Work out the finished part from the listing and answer in its coordinate system (mm). Face numbers are marked on the shaded views. Coordinates: 2 decimals unless noted, no trailing zeros. Write each loop counter-clockwise with the first axis right and the second up, starting at its lowest first coordinate (ties: lowest second). Pieces come first, ordered by that corner, then holes. Notation, with made-up numbers: (-21, 3) - (8, 3) arc R24 ccw to (8, 15) - close; hole circle Ø9 at (66, 36.25). An arc over 180 degrees is marked (long way). Use one line per item in the form item = value. Start each with the question number.
Item 1: Consider probe 1 along Z at (x, y) = (45.25, 0); probe 2 along Z at (x, y) = (21.5, 0); probe 3 along X at (y, z) = (7, 34). Determine where each line is inside the solid, lowest interval first.
Item 2: A cutting plane is placed at A-A (z = -2). Write down the section's boundary in (x, y), then the cut area to 3 significant figures.
Item 3: A cutting plane is placed at D-D (y = 8). Write down the section's boundary in (x, z).
Item 4: A cutting plane is placed at C-C (x = -40). Write down the section's boundary in (y, z).
Item 5: A cutting plane is placed at B-B (y = 0). Write down the section's boundary in (x, z), then the cut area to 3 significant figures.
Item 6: Determine the mould class of the marked faces 1, 2 and 3 for opening direction X: released by +X, released by -X, zero draft, split by the parting line, or undercut.
Item 7: Given pin 1 (3 mm diameter, centred on x = 37, z = 7, fed in from -Y); pin 2 (1.5 mm diameter, centred on x = -20, z = 0, fed in from +Y); pin 3 (5 mm diameter, centred on x = 15, y = 10, fed in from +Z); pin 4 (8 mm diameter, centred on y = 0, z = 34.76, fed in from -X) (1 decimal), each flat-ended and moving along its own axis, determine where each tip first touches the part or whether it passes through.
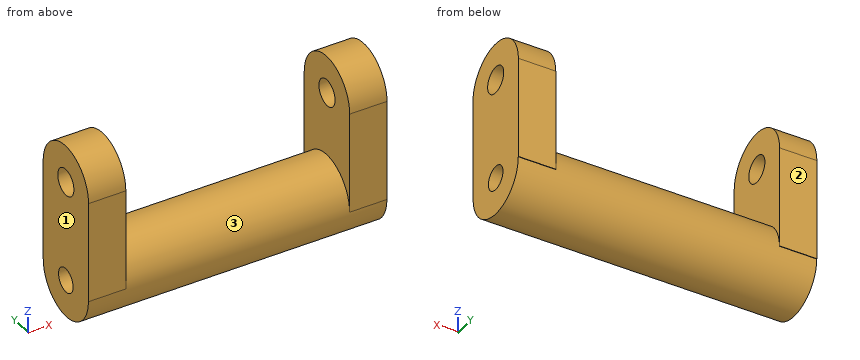
from build123d import *

# Parameters (mm, degrees)
F0_R     = 12.7485465516
F2_DEPTH = 50.8
F4_DEPTH = 50.8
F6_DEPTH = 38.1
F7_DEPTH = 50.8
F8_R     = 4.5528503381
F8_R_2   = 4.1100274938
F9_DEPTH = 101.601


with BuildPart() as f2:
    # F0 (on Right) → F2 (new body)
    with BuildSketch(Plane.YZ):
        Circle(F0_R)
    extrude(amount=F2_DEPTH)

    # F3: F2 across plane


with BuildPart() as f2_1:
    add(f2.part)
    add(f2.part.mirror(Plane.YZ))

    # F1 (on Right) → F4 (join)
    with BuildSketch(Plane.YZ):
        with BuildLine():
            Line((-12.815132901, 34.7624458373), (12.815132901, 34.7624458373))
            ThreePointArc((12.815132901, 34.7624458373), (0, 47.5775787383), (-12.815132901, 34.7624458373))
        make_face()
        with BuildLine():
            Line((12.8961233422, 34.7624458373), (12.815132901, 34.7624458373))
            ThreePointArc((12.815132901, 34.7624458373), (0, 21.9473129363), (-12.815132901, 34.7624458373))
            Line((-12.815132901, 34.7624458373), (-12.815132901, 0))
            Line((-12.815132901, 0), (12.8961233422, 0))
            Line((12.8961233422, 0), (12.8961233422, 34.7624458373))
        make_face()
        with BuildLine():
            ThreePointArc((-12.815132901, 34.7624458373), (0, 21.9473129363), (12.815132901, 34.7624458373))
            Line((12.815132901, 34.7624458373), (-12.815132901, 34.7624458373))
        make_face()
    extrude(amount=F4_DEPTH)

    # F5: F2 across plane


with BuildPart() as f2_2:
    add(f2_1.part)
    add(f2_1.part.mirror(Plane.YZ))

    # F1 (on Right) → F6 (cut, symmetric)
    with BuildSketch(Plane.YZ):
        with BuildLine():
            Line((-12.815132901, 34.7624458373), (12.815132901, 34.7624458373))
            ThreePointArc((12.815132901, 34.7624458373), (0, 47.5775787383), (-12.815132901, 34.7624458373))
        make_face()
        with BuildLine():
            Line((12.8961233422, 34.7624458373), (12.815132901, 34.7624458373))
            ThreePointArc((12.815132901, 34.7624458373), (0, 21.9473129363), (-12.815132901, 34.7624458373))
            Line((-12.815132901, 34.7624458373), (-12.815132901, 0))
            Line((-12.815132901, 0), (12.8961233422, 0))
            Line((12.8961233422, 0), (12.8961233422, 34.7624458373))
        make_face()
        with BuildLine():
            ThreePointArc((-12.815132901, 34.7624458373), (0, 21.9473129363), (12.815132901, 34.7624458373))
            Line((12.815132901, 34.7624458373), (-12.815132901, 34.7624458373))
        make_face()
    extrude(amount=F6_DEPTH, both=True, mode=Mode.SUBTRACT)

    # F0 (on Right) → F7 (join, symmetric)
    with BuildSketch(Plane.YZ):
        Circle(F0_R)
    extrude(amount=F7_DEPTH, both=True)

    # F8 (on face) → F9 (cut, through all)
    with BuildSketch(Plane.YZ.offset(50.8)):
        with Locations((0, 34.7624458373)):
            Circle(F8_R)
        Circle(F8_R_2)
    extrude(amount=-F9_DEPTH, mode=Mode.SUBTRACT)


solid = f2_2.part
Answer:
q1.probe_1 = -12.75 to -4.11, 4.11 to 30.21, 39.32 to 47.58
q1.probe_2 = -12.75 to -4.11, 4.11 to 12.75
q1.probe_3 = -50.8 to -38.1, 38.1 to 50.8
q2.outline = (-50.8, -12.59) - (50.8, -12.59) - (50.8, -3.59) - (-50.8, -3.59) - close; (-50.8, 3.59) - (50.8, 3.59) - (50.8, 12.59) - (-50.8, 12.59) - close
q2.area = 1,830 mm²
q3.outline = (-50.8, -9.93) - (50.8, -9.93) - (50.8, 44.77) - (38.1, 44.77) - (38.1, 9.93) - (-38.1, 9.93) - (-38.1, 44.77) - (-50.8, 44.77) - close
q4.outline = (-12.82, 0) - (-12.75, 0) arc R12.75 ccw to (12.75, 0) - (12.9, 0) - (12.9, 34.76) - (12.82, 34.76) arc R12.82 ccw to (-12.82, 34.76) - close; hole circle Ø9.11 at (0, 34.76); hole circle Ø8.22 at (0, 0)
q5.outline = (-50.8, -12.75) - (50.8, -12.75) - (50.8, -4.11) - (-50.8, -4.11) - close; (-50.8, 4.11) - (50.8, 4.11) - (50.8, 30.21) - (38.1, 30.21) - (38.1, 12.75) - (-38.1, 12.75) - (-38.1, 30.21) - (-50.8, 30.21) - close; (-50.8, 39.32) - (-38.1, 39.32) - (-38.1, 47.58) - (-50.8, 47.58) - close; (38.1, 39.32) - (50.8, 39.32) - (50.8, 47.58) - (38.1, 47.58) - close
q5.area = 2,410 mm²
q6.face_1 = released by -X
q6.face_2 = zero draft
q6.face_3 = undercut
q7.pin_1 = -12.82
q7.pin_2 = 12.75
q7.pin_3 = 10.31
q7.pin_4 = through
